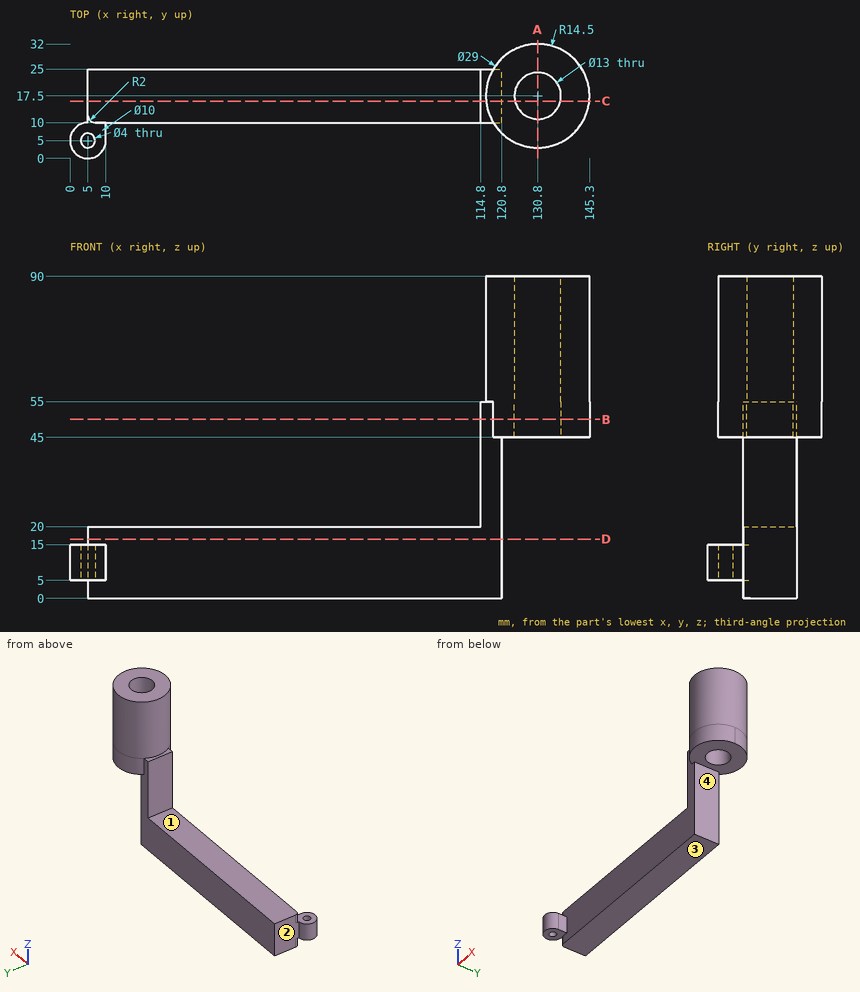
Geometry check sheet. Reference: drawing and pictorial views, mm from the part's lowest x, y, z. A direction names the side the tool comes from. Round coordinates to 2 decimals unless told otherwise and drop trailing zeros. Loops run counter-clockwise (first coordinate to the right, second up) from the corner with the lowest first, then second, coordinate; pieces in that order, holes last. Notation, with made-up numbers: (49.25, 14.5) - (61.25, 14.5) arc R37 cw to (61.25, 53.5) - close; hole circle Ø10 at (-22.5, -33.5). An arc over 180 degrees is marked (long way). One line per question, with ' | ' between items. Start each with the question number.
1. Cross-section at D-D on z = 16.5. Record the cut outline in (x, y).
2. Cross-section at A-A on x = 130.8. Record the cut outline in (y, z).
3. Depth check by flat-ended pin: pin 1 (1.5 mm diameter, centred on x = 47, y = 17, fed in from +Z); pin 2 (5.5 mm diameter, centred on y = 7, z = 12.5, fed in from +X); pin 3 (16.5 mm diameter, centred on y = 14.5, z = 10, fed in from -X); pin 4 (10 mm diameter, centred on x = 30, y = 15, fed in from -Z). Enter the tip coordinate at first touch or a pass-through.
4. Cross-section at C-C on y = 16. Record the cut outline in (x, z).
5. Tool access check on the marked faces 1, 2, 3 and 4. Record the directions out of +Z, -Z, +X, -X, +Y, -Y that give a thin tool (end or side, any length) a straight path to the whole face; none if there is none.
6. Cross-section at B-B on z = 50. Record the cut outline in (x, y).
7. Scan lines: line 1 (X direction, y = 17, z = 78); line 2 (Z direction, x = 12, y = 23); line 3 (Y direction, x = 130, z = 50). Record each from-to range of solid material in increasing order. Write a range as [from, to].
Taken from the geometry:
1) outline: (5, 12) arc R2 ccw to (7, 10) - (120.8, 10) - (120.8, 25) - (5, 25) - close
2) outline: (3, 45) - (11, 45) - (11, 90) - (3, 90) - close; (24, 45) - (32, 45) - (32, 90) - (24, 90) - close
3) pin 1: z = 20 | pin 2: x = 10 | pin 3: x = 0.16 | pin 4: z = 0
4) outline: (5, 0) - (120.8, 0) - (120.8, 45) - (124.48, 45) - (124.48, 90) - (116.38, 90) - (116.38, 55) - (114.8, 55) - (114.8, 20) - (5, 20) - close; (137.12, 45) - (145.22, 45) - (145.22, 90) - (137.12, 90) - close
5) face 1: +Z, -X, +Y, -Y | face 2: +Z, -Z, -X, +Y | face 3: -Z, +X, -X, +Y, -Y | face 4: -Z, +X, +Y, -Y
6) outline: (114.8, 10) - (118.39, 10) arc R14.5 ccw (long way) to (118.39, 25) - (114.8, 25) - close; hole circle Ø13 at (130.8, 17.5)
7) line 1: [116.31, 124.32], [137.28, 145.29] | line 2: [0, 20] | line 3: [3.02, 11.05], [23.95, 31.98]
